Source: CAD feature listing. Evaluate the final solid. Frame: model axes, mm. Face numbers are marked on the shaded views. A direction names the side the tool comes from. Round coordinates to 2 decimals unless told otherwise and drop trailing zeros. Loops run counter-clockwise (first coordinate to the right, second up) from the corner with the lowest first, then second, coordinate; pieces in that order, holes last. Notation, with made-up numbers: M 25,43 L 33,43 A16 ccw 33,59 Z; hole C -37,38 d11. An arc over 180 degrees is marked long. Answer as a JSON object with one key per item and string values.
from build123d import *

# Parameters (mm, degrees)
SKETCH1_W                = 42.3
SKETCH1_H                = 42.3
BOSS_EXTRUDE1_DEPTH      = 33.5
SKETCH2_R                = 1.65
CUT_EXTRUDE1_DEPTH       = 10
SKETCH3_R                = 11
BOSS_EXTRUDE2_DEPTH      = 2
SKETCH4_R                = 2.5
BOSS_EXTRUDE3_DEPTH      = 22
BOSS_EXTRUDE3_DEPTH_BACK = 45
SKETCH5_W                = 21.3
SKETCH5_H                = 2.8
BOSS_EXTRUDE4_DEPTH      = 7.15
CHAMFER1_SIZE            = 5


with BuildPart() as part:
    # Sketch1 → Boss-Extrude1 (new body)
    with BuildSketch(Plane.XY):
        with Locations((21.15, 21.15)):
            Rectangle(SKETCH1_W, SKETCH1_H)
    extrude(amount=BOSS_EXTRUDE1_DEPTH)

    # Sketch2 → Cut-Extrude1 (cut)
    with BuildSketch(Plane.XY.offset(33.5)):
        with Locations((5.65, 36.65)):
            Circle(SKETCH2_R)
        with Locations((36.65, 36.65)):
            Circle(SKETCH2_R)
        with Locations((5.65, 5.65)):
            Circle(SKETCH2_R)
        with Locations((36.65, 5.65)):
            Circle(SKETCH2_R)
    extrude(amount=-CUT_EXTRUDE1_DEPTH, mode=Mode.SUBTRACT)

    # Sketch3 → Boss-Extrude2 (add)
    with BuildSketch(Plane.XY.offset(33.5)):
        with Locations((21.15, 21.15)):
            Circle(SKETCH3_R)
    extrude(amount=BOSS_EXTRUDE2_DEPTH)

    # Sketch4 → Boss-Extrude3 (add, two sides)
    with BuildSketch(Plane.XY.offset(35.5)) as boss_extrude3_sk:
        with Locations((21.15, 21.15)):
            Circle(SKETCH4_R)
    extrude(amount=BOSS_EXTRUDE3_DEPTH)
    extrude(boss_extrude3_sk.sketch, amount=-BOSS_EXTRUDE3_DEPTH_BACK)

    # Sketch5 → Boss-Extrude4 (add)
    with BuildSketch(Plane(origin=(0, 0, 0), x_dir=(-1, 0, 0), z_dir=(0, 0, -1))):
        with Locations((-21.15, -1.4)):
            Rectangle(SKETCH5_W, SKETCH5_H)
    extrude(amount=-BOSS_EXTRUDE4_DEPTH)

    # Chamfer1
    chamfer1_edges = [part.edges().sort_by_distance(p)[0] for p in [
        (0, 0, 16.75),
        (42.3, 0, 16.75),
        (42.3, 42.3, 16.75),
        (0, 42.3, 16.75),
    ]]
    chamfer(chamfer1_edges, length=CHAMFER1_SIZE)


solid = part.part
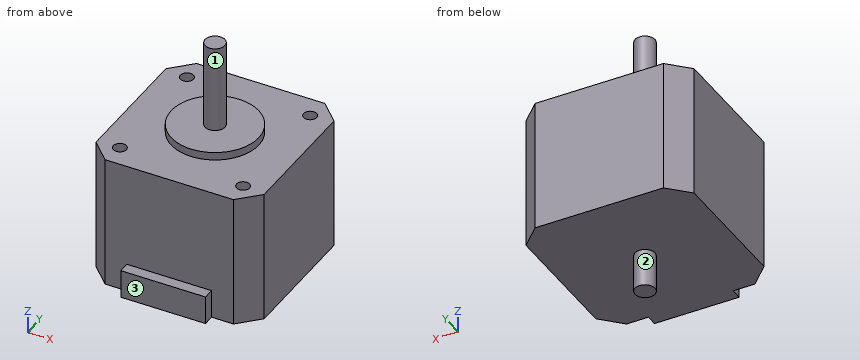
Item 1: Contact query for flat-ended pins moving along their axis: pin 1 Ø1.4 at (x, y) = (22.5, -0.5) entering from +Z; pin 2 Ø16 at (x, z) = (21.5, 18) entering from -Y; pin 3 Ø2 at (x, y) = (36.65, 5.65) entering from +Z. Output: stop coordinate, or through.
Answer sheet:
{"pin 1": "stops at z = 33.5", "pin 2": "stops at y = 0", "pin 3": "stops at z = 23.5"}
Item 2: Section A-A on x = 21.15. Return the cut outline in (y, z), then the cut area to 3 significant figures.
Answer sheet:
{"outline": "M -2.8,0 L 18.65,0 L 18.65,-9.5 L 23.65,-9.5 L 23.65,0 L 42.3,0 L 42.3,33.5 L 32.15,33.5 L 32.15,35.5 L 23.65,35.5 L 23.65,57.5 L 18.65,57.5 L 18.65,35.5 L 10.15,35.5 L 10.15,33.5 L 0,33.5 L 0,7.15 L -2.8,7.15 Z", "area": "1,640 mm²"}
Item 3: Access query for the marked faces 1, 2 and 3. Directions: +Z, -Z, +X, -X, +Y, -Y. A direction counts if a zero-diameter tool reaches every point of the face in a straight line with its end or side. Return the directions, or none.
Answer sheet:
{"face 1": "+Z", "face 2": "-Z", "face 3": "+Z, -Z, +X, -X, -Y"}
Item 4: Section B-B on z = 25. Return the cut outline in (x, y).
Answer sheet:
{"outline": "M 0,5 L 5,0 L 37.3,0 L 42.3,5 L 42.3,37.3 L 37.3,42.3 L 5,42.3 L 0,37.3 Z; hole C 5.65,5.65 d3.3; hole C 5.65,36.65 d3.3; hole C 36.65,5.65 d3.3; hole C 36.65,36.65 d3.3"}
Item 5: Section C-C on y = 25. Return the cut outline in (x, z), then the cut area to 3 significant figures.
Answer sheet:
{"outline": "M 0,0 L 42.3,0 L 42.3,33.5 L 31.45,33.5 L 31.45,35.5 L 10.85,35.5 L 10.85,33.5 L 0,33.5 Z", "area": "1,460 mm²"}
Item 6: Line query: probe 1 along Y at (x, z) = (36.65, 29.25); probe 2 along Y at (x, z) = (5, 28). Output: solid intervals per line, ascending. Write a range as from..to.
Answer sheet:
{"probe 1": "y = 0..4, 7.3..35, 38.3..42.3", "probe 2": "y = 0..4.13, 7.17..35.13, 38.17..42.3"}
Item 7: Section D-D on z = 51. Return the cut outline in (x, y).
Answer sheet:
{"outline": "C 21.15,21.15 d5"}
